```python
from build123d import *

# Parameters (mm, degrees)
F1_DEPTH = 12.7
F2_T     = -2.54
F3_R     = 1.5875418941
F4_DEPTH = 45.72


# Not quite as in the source:
# - a feature names something its author has since deleted; it is built from what else it names


with BuildPart() as f1:
    # F0 (on Front) → F1 (new body)
    with BuildSketch(Plane.XZ):
        Polygon((-105.322439312, 88.9), (-105.322439312, -12.7), (-98.972439312, -12.7), (-98.972439312, 0), (-98.972439312, 82.55), (-60.872439312, 82.55), (-60.872439312, 0), (-60.872439312, -12.7), (-54.522439312, -12.7), (-54.522439312, 88.9), align=None)
    extrude(amount=F1_DEPTH)

    # F2
    f2_openings = [f1.faces().sort_by_distance(p)[0] for p in [
        (-60.872439, -6.35, 34.925),
        (-79.922439, -6.35, 82.55),
        (-98.972439, -6.35, 34.925),
    ]]
    offset(amount=F2_T, openings=f2_openings)

    # F3 (on face) → F4 (join)
    with BuildSketch(Plane(origin=(-57.062439312, 0, 0), x_dir=(0, -1, 0), z_dir=(-1, 0, 0))):
        with Locations((6.2330360524, 0)):
            Circle(F3_R)
    extrude(amount=F4_DEPTH)


solid = f1.part
```
The listing builds one solid part. Answer for the finished solid, in the listing's coordinates (mm). A direction names the side the tool comes from. Give positions to 0.01 mm unless a question says otherwise; leave off trailing zeros. Loops run counter-clockwise (first coordinate to the right, second up) from the corner with the lowest first, then second, coordinate; pieces in that order, holes last. Notation, with made-up numbers: (0.5, 69.25) - (5.5, 69.25) arc R10 ccw to (5.5, 76.25) - close; hole circle Ø11 at (3.5, 81). An arc over 180 degrees is marked (long way). Return JSON: item names as keys, results as strings. Group by question number.
1. Given pin 1 Ø6 at (x, y) = (-79.5, -7) entering from -Z; pin 2 Ø0.8 at (x, y) = (-81.5, -1.5) entering from -Z; pin 3 Ø13.5 at (x, z) = (-88.5, 40.5) entering from +Y; pin 4 Ø1 at (x, y) = (-84, -3.5) entering from -Z, each flat-ended and moving along its own axis, determine where each tip first touches the part or whether it passes through.
2. Find section D-D (z = 0). Write down the section's boundary in (x, y).
3. Determine the mould class of faces 1 (the flat face through (-80, -1, 82.55)), 2 (the flat face through (-58, -6, -12.7)), 3 (the flat face through (-54.522, -6, 37)) for opening direction X: pulls with the +X half, pulls with the -X half, needs draft (parallel to the pull), parting line crosses it, or undercut.
4. Which of the six approach directions +Z, -Z, +X, -X, +Y, -Y give full straight-line access (tool end or side, diameter ignored) to faces 4 (the flat face through (-80, -11, 82.55)), 5 (the flat face through (-101, -12.7, 50)), 6 (the flat face through (-100, -2.54, 45))?
5. Find section A-A (x = -58.5). Write down the section's boundary in (y, z).
6. Straight lines are drawn through the part: line 1 (Z direction, x = -101, y = -6.5); line 2 (Z direction, x = -94.5, y = -6.5); line 3 (X direction, y = -1.5, z = 76). For each, find the intervals that lie inside material, in ascending order. Write a range as [from, to].
7. Find section B-B (z = 54). Write down the section's boundary in (x, y).
8. Find section C-C (x = -96). Write down the section's boundary in (y, z), then the cut area to 3 significant figures.
Verdict:
{
 "1": {"pin 1": "stops at z = -1.59", "pin 2": "stops at z = 82.55", "pin 3": "passes through", "pin 4": "stops at z = 86.36"},
 "2": {"outline": "(-105.32, -12.7) - (-98.97, -12.7) - (-98.97, -10.16) - (-102.78, -10.16) - (-102.78, -7.82) - (-57.06, -7.82) - (-57.06, -10.16) - (-60.87, -10.16) - (-60.87, -12.7) - (-54.52, -12.7) - (-54.52, 0) - (-60.87, 0) - (-60.87, -2.54) - (-57.06, -2.54) - (-57.06, -4.65) - (-102.78, -4.65) - (-102.78, -2.54) - (-98.97, -2.54) - (-98.97, 0) - (-105.32, 0) - close"},
 "3": {"face 1": "undercut", "face 2": "needs draft", "face 3": "pulls with the +X half"},
 "4": {"face 4": "-Z, +Y, -Y", "face 5": "+Z, -Z, +X, -X, -Y", "face 6": "none"},
 "5": {"outline": "(-12.7, -12.7) - (0, -12.7) - (0, 88.9) - (-12.7, 88.9) - close; circle Ø3.18 at (-6.23, 0); hole (-10.16, -10.16) - (-2.54, -10.16) - (-2.54, 86.36) - (-10.16, 86.36) - close"},
 "6": {"line 1": "z = [-12.7, -10.16], [-1.56, 1.56], [86.36, 88.9]", "line 2": "z = [-1.56, 1.56], [86.36, 88.9]", "line 3": "x = [-105.32, -98.97], [-60.87, -54.52]"},
 "7": {"outline": "(-105.32, -12.7) - (-98.97, -12.7) - (-98.97, -10.16) - (-102.78, -10.16) - (-102.78, -2.54) - (-98.97, -2.54) - (-98.97, 0) - (-105.32, 0) - close; (-60.87, -12.7) - (-54.52, -12.7) - (-54.52, 0) - (-60.87, 0) - (-60.87, -2.54) - (-57.06, -2.54) - (-57.06, -10.16) - (-60.87, -10.16) - close"},
 "8": {"outline": "(-12.7, 82.55) - (-10.16, 82.55) - (-10.16, 86.36) - (-2.54, 86.36) - (-2.54, 82.55) - (0, 82.55) - (0, 88.9) - (-12.7, 88.9) - close; circle Ø3.18 at (-6.23, 0)", "area": "59.5 mm^2"}
}
